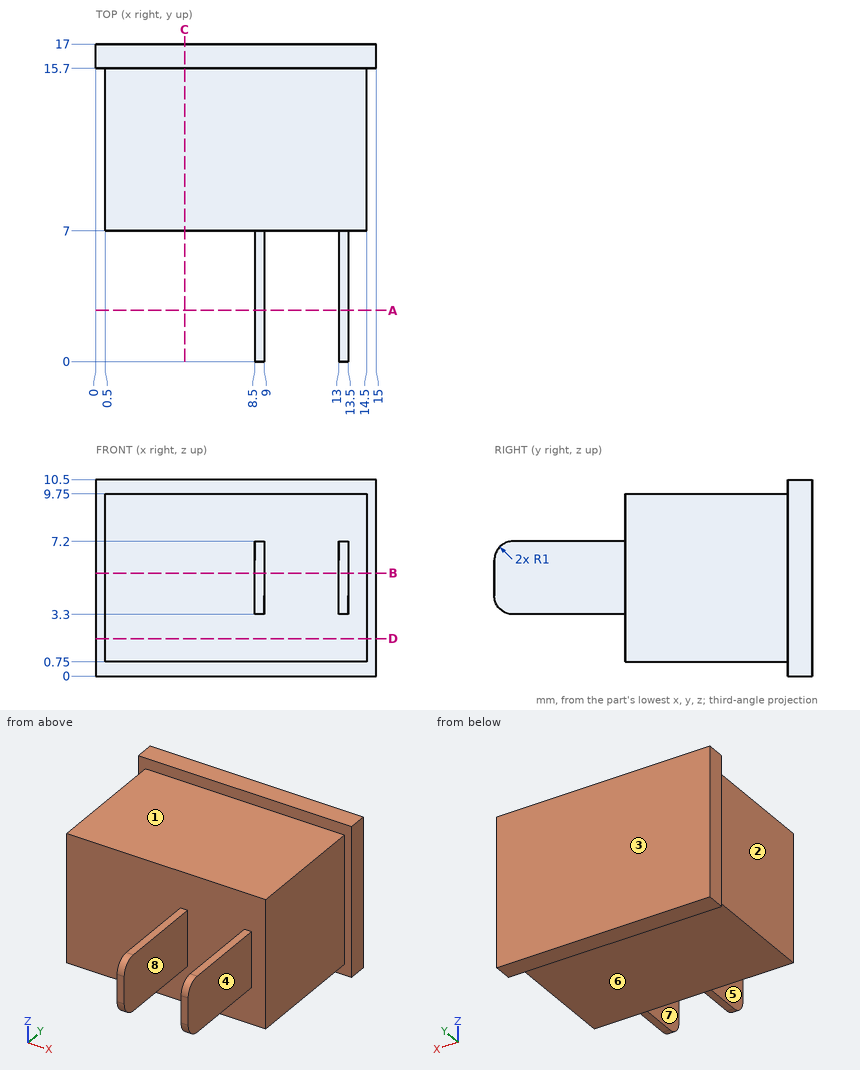
Design review of the part shown in the three views and the two pictorial views. Dimensions are in mm from the part's minimum x, y and z. A direction names the side the tool comes from. Coordinates: 2 decimals unless noted, no trailing zeros. Loops run counter-clockwise (first coordinate to the right, second up) from the corner with the lowest first, then second, coordinate; pieces in that order, holes last. Notation, with made-up numbers: (76.5, -16.5) - (86.5, -16.5) arc R36 ccw to (86.5, 18.5) - close; hole circle Ø3 at (60.25, 25.5). An arc over 180 degrees is marked (long way). Use a Markdown table: item, result. Add a question column.
Item 1: We need section A-A (y = 2.75). Give the boundary of the cut face in (x, z), and give its area (3 significant figures).
Item 2: We need section C-C (x = 4.75). Give the boundary of the cut face in (y, z).
Item 3: We need section D-D (z = 2). Give the boundary of the cut face in (x, y).
Item 4: For line 1 (X direction, y = 1.5, z = 6.25); line 2 (Y direction, x = 13.75, z = 1); line 3 (Z direction, x = 3.5, y = 10.5), list the stretches that pass through material, from the lowest coordinate up.
Item 5: Mouldability with a two-part tool opening along X and no side actions: class the marked faces 5, 6, 7 and 8 as pulls with the +X half, pulls with the -X half, needs draft (parallel to the pull), parting line crosses it, or undercut.
Item 6: Insertion check: pin 1 Ø5 at (x, y) = (10.5, 11) entering from -Z; pin 2 Ø3 at (y, z) = (3.5, 5) entering from -X; pin 3 Ø5 at (x, z) = (3.5, 7.5) entering from -Y. Each pin has a flat end and moves straight along its axis. Give the tip position at first contact, or say it passes through.
Item 7: We need section B-B (z = 5.5). Give the boundary of the cut face in (x, y).
Item 8: Tool access review of the marked faces 1, 2, 3 and 4: name each direction out of +Z, -Z, +X, -X, +Y, -Y from which nothing blocks a thin tool from reaching the whole face with its end or side.
Results list:
| question | item | result |
|---|---|---|
| 1 | outline | (8.5, 3.3) - (9, 3.3) - (9, 7.2) - (8.5, 7.2) - close; (13, 3.3) - (13.5, 3.3) - (13.5, 7.2) - (13, 7.2) - close |
| 1 | area | 3.90 mm^2 |
| 2 | outline | (7, 0.75) - (15.7, 0.75) - (15.7, 0) - (17, 0) - (17, 10.5) - (15.7, 10.5) - (15.7, 9.75) - (7, 9.75) - close |
| 3 | outline | (0, 15.7) - (0.5, 15.7) - (0.5, 7) - (14.5, 7) - (14.5, 15.7) - (15, 15.7) - (15, 17) - (0, 17) - close |
| 4 | line 1 | x = 8.5 to 9, 13 to 13.5 |
| 4 | line 2 | y = 7 to 17 |
| 4 | line 3 | z = 0.75 to 9.75 |
| 5 | face 5 | pulls with the -X half |
| 5 | face 6 | needs draft |
| 5 | face 7 | undercut |
| 5 | face 8 | undercut |
| 6 | pin 1 | stops at z = 0.75 |
| 6 | pin 2 | stops at x = 8.5 |
| 6 | pin 3 | stops at y = 7 |
| 7 | outline | (0, 15.7) - (0.5, 15.7) - (0.5, 7) - (8.5, 7) - (8.5, 0) - (9, 0) - (9, 7) - (13, 7) - (13, 0) - (13.5, 0) - (13.5, 7) - (14.5, 7) - (14.5, 15.7) - (15, 15.7) - (15, 17) - (0, 17) - close |
| 8 | face 1 | +Z, +X, -X, -Y |
| 8 | face 2 | +Z, -Z, -X, -Y |
| 8 | face 3 | +Z, -Z, +X, -X, +Y |
| 8 | face 4 | +Z, -Z, +X, -Y |
